Can you work these out from the drawing? Everything is in mm from the part's minimum corner. A direction names the side the tool comes from. Coordinates: 2 decimals unless noted, no trailing zeros. Order: outer loops, then holes, each group sorted by start corner. A loop starts at its lowest first (then second) coordinate and runs counter-clockwise, first axis right, second up. Notation, with made-up numbers: (30.5, -11.75) -> (53.5, -11.75) arc R16 cw to (53.5, -2.75) -> close; hole circle Ø1 at (77, 75). An arc over 180 degrees is marked (long way). Use a Markdown table: item, result. Add a question column.
1) Thinking about a two-plate mould opening in Y: for the marked faces 5, 6 and 7, which applies, +Y half, -Y half, draft (parallel to the pull), parting line (faces both ways), or undercut?
2) If I drill on L1, parallel to Y at x = 3.2, z = 25 (1 decimal); L2, parallel to Z at x = 1.35, y = 55; L3, parallel to Y at x = 3.4, z = 7, over which ranges is the centre line in solid material (lowest first)? Write a range as [from, to].
3) If we section it at B-B (z = 13.75): Write out the boundary of the cut face in (x, y), plus the area to 3 significant figures.
4) If we section it at C-C (y = 25.5): Write out the boundary of the cut face in (x, z), plus the area to 3 significant figures.
5) Will these pins go through, and if not, where does the flat tip stop? pin 1 Ø2.5 at (x, y) = (2.5, 11.5) entering from +Z; pin 2 Ø2 at (y, z) = (38, 4) entering from -X.
6) Which directions (+Z, -Z, +X, -X, +Y, -Y) give clear straight access to the entire face, cutting with the end or side of a thin tool? Please do the marked faces 1, 2, 3 and 4.
7) If we section it at A-A (x = 2.15): Write out the boundary of the cut face in (y, z) (1 decimal).
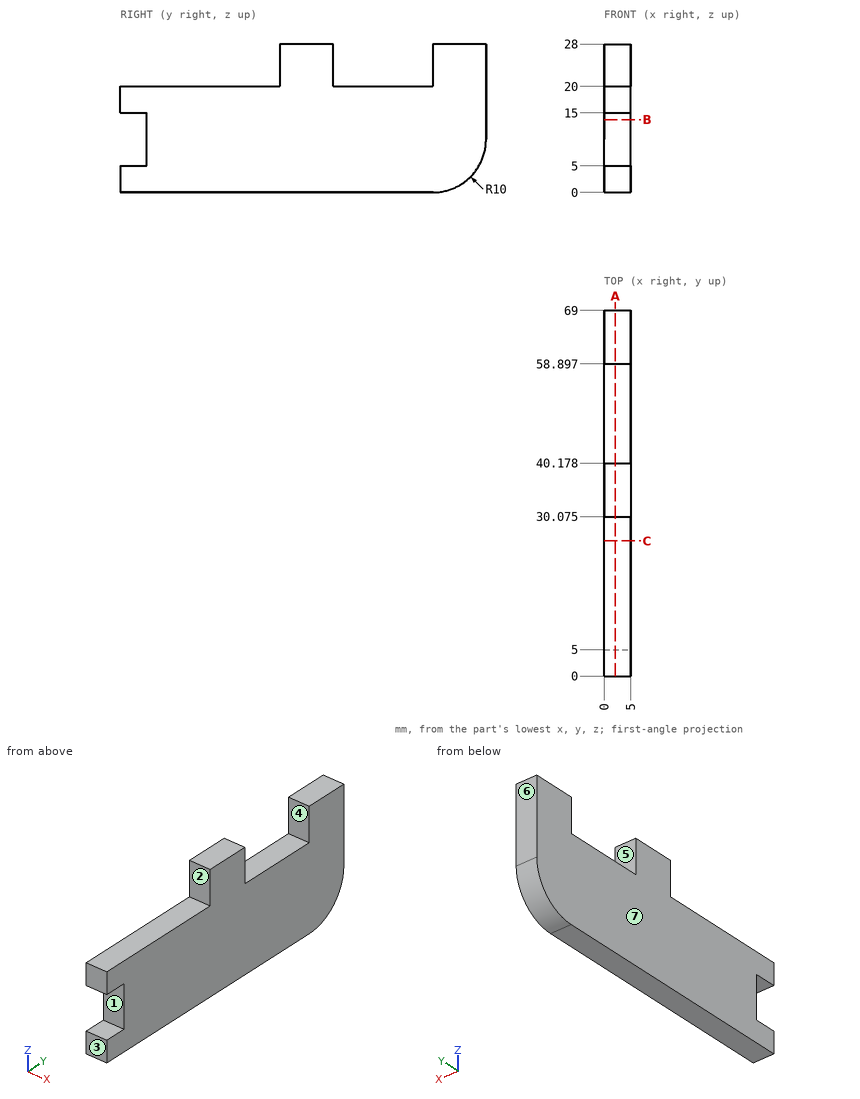
Answer sheet:
| question | item | result |
|---|---|---|
| 1 | face 5 | undercut |
| 1 | face 6 | +Y half |
| 1 | face 7 | draft |
| 2 | L1 | [30.1, 40.2], [58.9, 69] |
| 2 | L2 | [0, 20] |
| 2 | L3 | [5, 68.54] |
| 3 | outline | (0, 5) -> (5, 5) -> (5, 69) -> (0, 69) -> close |
| 3 | area | 320 mm2 |
| 4 | outline | (0, 0) -> (5, 0) -> (5, 20) -> (0, 20) -> close |
| 4 | area | 100 mm2 |
| 5 | pin 1 | z = 20 |
| 5 | pin 2 | x = 0 |
| 6 | face 1 | +X, -X, -Y |
| 6 | face 2 | +Z, +X, -X, -Y |
| 6 | face 3 | +Z, -Z, +X, -X, -Y |
| 6 | face 4 | +Z, +X, -X |
| 7 | outline | (0, 0) -> (59, 0) arc R10 ccw to (69, 10) -> (69, 28) -> (58.9, 28) -> (58.9, 20) -> (40.2, 20) -> (40.2, 28) -> (30.1, 28) -> (30.1, 20) -> (0, 20) -> (0, 15) -> (5, 15) -> (5, 5) -> (0, 5) -> close |
